The drawing under review shows one solid part. Ordinate dimensions are in mm from its lowest x, y, z. Give positions to 0.01 mm unless a question says otherwise; leave off trailing zeros. Loops run counter-clockwise (first coordinate to the right, second up) from the corner with the lowest first, then second, coordinate; pieces in that order, holes last.
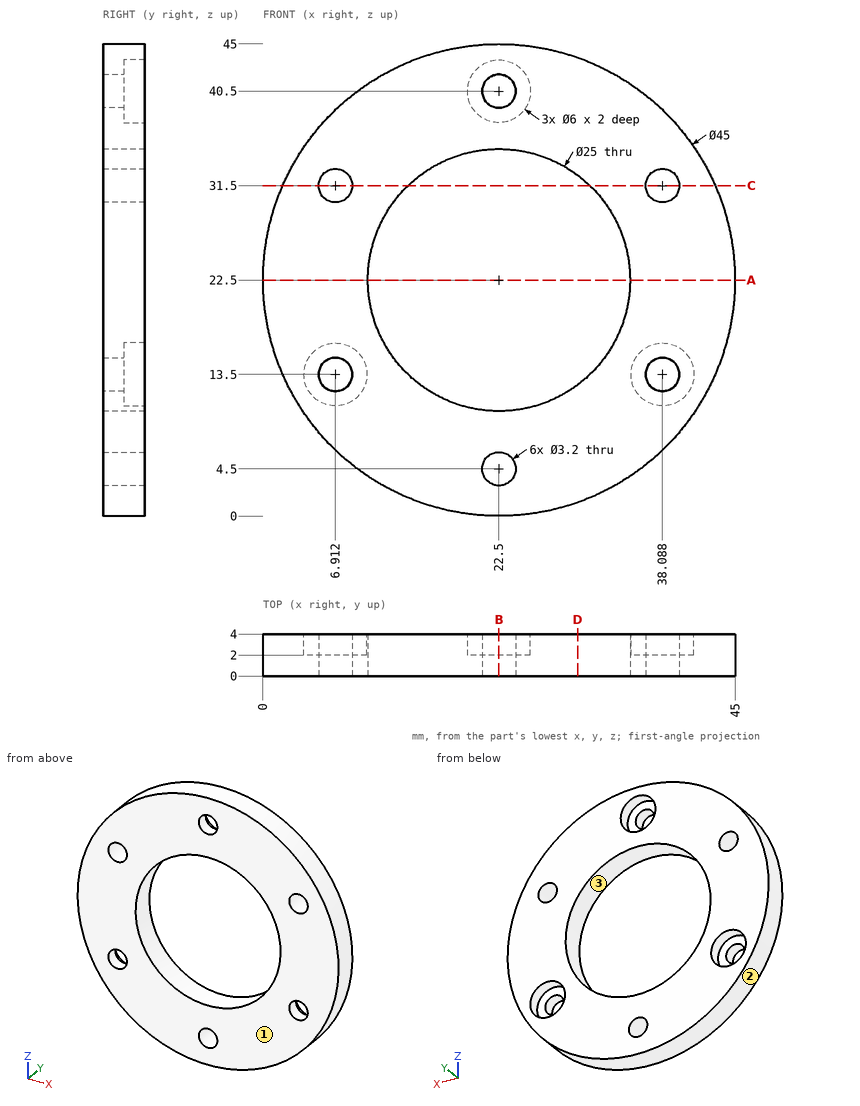
Item 1: Take a section at D-D on x = 30. Give the boundary of the cut face in (y, z).
Answer:
outline: (0, 1.29) - (4, 1.29) - (4, 12.5) - (0, 12.5) - close; (0, 32.5) - (4, 32.5) - (4, 43.71) - (0, 43.71) - close
Item 2: Clearance check with flat-ended pins moving along their axes: pin 1 Ø3 at (x, z) = (7, 14) entering from +Y; pin 2 Ø1 at (y, z) = (2.5, 30.5) entering from -X; pin 3 Ø8 at (x, z) = (38.09, 13.5) entering from -Y; pin 4 Ø1 at (y, z) = (2.5, 39) entering from -X. State where each tip first meets the part, or that it passes through.
Answer:
pin 1: stops at y = 2
pin 2: stops at x = 1.29
pin 3: stops at y = 0
pin 4: stops at x = 6.68
Item 3: The part is to be moulded in two halves that separate along X. For the marked faces 1, 2 and 3, say which applies: released by +X, released by -X, zero draft, split by the parting line, or undercut.
Answer:
face 1: zero draft
face 2: split by the parting line
face 3: undercut
Item 4: Take a section at A-A on z = 22.5. Give the boundary of the cut face in (x, y).
Answer:
outline: (0, 0) - (10, 0) - (10, 4) - (0, 4) - close; (35, 0) - (45, 0) - (45, 4) - (35, 4) - close
Item 5: Take a section at C-C on z = 31.5. Give the boundary of the cut face in (x, y) (1 decimal).
Answer:
outline: (1.9, 0) - (5.3, 0) - (5.3, 4) - (1.9, 4) - close; (8.5, 0) - (13.8, 0) - (13.8, 4) - (8.5, 4) - close; (31.2, 0) - (36.5, 0) - (36.5, 4) - (31.2, 4) - close; (39.7, 0) - (43.1, 0) - (43.1, 4) - (39.7, 4) - close
Item 6: For L1, parallel to X at y = 1.45, z = 13.5 (1 decimal); L2, parallel to Z at x = 20.5, y = 2.15 (1 decimal); L3, parallel to Z at x = 22, y = 3.5 (1 decimal), list the stretches that pass through material, from the lowest coordinate up.
Answer:
L1: x = 1.9 to 5.3, 8.5 to 13.8, 31.2 to 36.5, 39.7 to 43.1
L2: z = 0.1 to 10.2, 34.8 to 38.3, 42.7 to 44.9
L3: z = 0 to 3, 6 to 10, 35 to 37.5, 43.5 to 45
Item 7: Take a section at B-B on x = 22.5. Give the boundary of the cut face in (y, z).
Answer:
outline: (0, 0) - (4, 0) - (4, 2.9) - (0, 2.9) - close; (0, 6.1) - (4, 6.1) - (4, 10) - (0, 10) - close; (0, 35) - (4, 35) - (4, 37.5) - (2, 37.5) - (2, 38.9) - (0, 38.9) - close; (0, 42.1) - (2, 42.1) - (2, 43.5) - (4, 43.5) - (4, 45) - (0, 45) - close
